Could you check a few things on this model? Use its own coordinates, in mm. A direction names the side the tool comes from. Give positions to 0.01 mm unless a question says otherwise; leave off trailing zeros. Write each loop counter-clockwise with the first axis right and the second up, starting at its lowest first coordinate (ties: lowest second). Pieces come first, ordered by that corner, then holes. Notation, with made-up numbers: M -19.5,26 L 13.5,26 A22 cw 13.5,48 Z; hole C 63,46.25 d11. An arc over 180 degrees is marked long. Use one line per item in the form item = value.
from build123d import *

# Parameters (mm, degrees)
SKETCH1_W           = 22.86
SKETCH1_H           = 22.86
BOSS_EXTRUDE1_DEPTH = 1.27
SKETCH3_W           = 22.86
SKETCH3_H           = 1.27
BOSS_EXTRUDE2_DEPTH = 47.593039283
SKETCH4_R           = 4
CUT_EXTRUDE2_DEPTH  = 10
SKETCH5_R           = 4
SKETCH5_W           = 8
SKETCH5_H           = 10.275395712
CUT_EXTRUDE3_DEPTH  = 2.54
SCALE2_SCALE        = 2.1


with BuildPart() as part:
    # Sketch1 → Boss-Extrude1 (new body)
    with BuildSketch(Plane(origin=(0, 0, 0), x_dir=(1, 0, 0), z_dir=(0, 1, 0))):
        with Locations((0.164586144, 0.124003255)):
            Rectangle(SKETCH1_W, SKETCH1_H)
    extrude(amount=BOSS_EXTRUDE1_DEPTH)

    # Sketch3 → Boss-Extrude2 (add)
    with BuildSketch(Plane.XZ):
        with Locations((0.164586144, -10.919003255)):
            Rectangle(SKETCH3_W, SKETCH3_H)
    extrude(amount=-BOSS_EXTRUDE2_DEPTH)

    # Sketch4 → Cut-Extrude2 (cut)
    with BuildSketch(Plane(origin=(0, 1.27, 0), x_dir=(1, 0, 0), z_dir=(0, 1, 0))):
        with Locations(Location((0, 0, 0), (0, 0, 270))):
            Circle(SKETCH4_R)
    extrude(amount=-CUT_EXTRUDE2_DEPTH, mode=Mode.SUBTRACT)

    # Sketch5 → Cut-Extrude3 (cut)
    with BuildSketch(Plane.XY.offset(-10.284003255)):
        with Locations((0.082545716, 37.799520725)):
            Circle(SKETCH5_R)
        with Locations((0.034649226, 27.524125013)):
            Circle(SKETCH5_R)
        with Locations((0.082545716, 32.661822869)):
            Rectangle(SKETCH5_W, SKETCH5_H)
        with BuildLine():
            ThreePointArc((4.034649226, 27.524125013), (0.344153636, 31.512132914), (-3.917454284, 28.141278028))
            Line((-3.917454284, 28.141278028), (-3.917454284, 27.524125013))
            Line((-3.917454284, 27.524125013), (4.034649226, 27.524125013))
        make_face()
        with BuildLine():
            Line((-3.917454284, 27.524125013), (-3.917454284, 28.141278028))
            ThreePointArc((-3.917454284, 28.141278028), (-0.274855184, 23.536117112), (4.034649226, 27.524125013))
            Line((4.034649226, 27.524125013), (-3.917454284, 27.524125013))
        make_face()
        with Locations((0, 10.961912138)):
            Circle(SKETCH5_R)
        with BuildLine():
            ThreePointArc((4.082545716, 37.799520725), (0.082545716, 41.799520725), (-3.917454284, 37.799520725))
            Line((-3.917454284, 37.799520725), (4.082545716, 37.799520725))
        make_face()
        with BuildLine():
            Line((4.082545716, 37.799520725), (-3.917454284, 37.799520725))
            ThreePointArc((-3.917454284, 37.799520725), (0.082545716, 33.799520725), (4.082545716, 37.799520725))
        make_face()
    extrude(amount=-CUT_EXTRUDE3_DEPTH, mode=Mode.SUBTRACT)


with BuildPart() as part_1:
    # Scale2: scaled about (0, 0, 0)
    add(part.part.scale(SCALE2_SCALE))


solid = part_1.part
1) If I drill on L1, parallel to Y at x = 0, z = -23; L2, parallel to X at y = 0.85, z = 0; L3, parallel to Z at x = 9.5, y = 9, over which ranges is the centre line in solid material (lowest first)?
Checked values:
L1 = 0 to 14.62, 31.42 to 49.4, 87.78 to 99.95
L2 = -23.66 to -8.4, 8.4 to 24.35
L3 = -24.26 to -21.6
2) For faces 1 (the flat face through (-8.227, 69, -23)), 2 (the flat face through (5.3, 50.6, -21.596)), 3 (the flat face through (0, 1, 23.743)), which set-ups out of +Z, -Z, +X, -X, +Y, -Y let a thin tool reach every point of the face, with its end or its side?
Checked values:
face_1 = +Z, -Z
face_2 = +Z, +X, -X, +Y
face_3 = +Z, +X, -X, +Y, -Y
3) I want a section at D-D, the plane x = -15.5. Please give me the cut outline in (y, z).
Checked values:
outline = M 0,-24.26 L 99.95,-24.26 L 99.95,-21.6 L 2.67,-21.6 L 2.67,23.74 L 0,23.74 Z
4) I want a section at C-C, the plane x = 0. Please give me the cut outline in (y, z), plus the area to 3 significant figures.
Checked values:
outline = M 0,-24.26 L 14.62,-24.26 L 14.62,-21.6 L 2.67,-21.6 L 2.67,-8.4 L 0,-8.4 Z; M 0,8.4 L 2.67,8.4 L 2.67,23.74 L 0,23.74 Z; M 31.42,-24.26 L 49.4,-24.26 L 49.4,-21.6 L 31.42,-21.6 Z; M 87.78,-24.26 L 99.95,-24.26 L 99.95,-21.6 L 87.78,-21.6 Z
area = 196 mm2
5) For pin 1 Ø10 at (x, z) = (-15, -9) entering from +Y; pin 2 Ø6 at (x, y) = (5.5, 71.5) entering from -Z; pin 3 Ø24 at (x, y) = (3, 48.5) entering from +Z, each with a flat end and sliding along its axis, tell me the tip position at first contact or that it passes through.
Checked values:
pin_1 = 2.67
pin_2 = through
pin_3 = -21.6
6) Thinking about a two-plate mould opening in Y: for faces 4 (the flat face through (0, 2.667, -9)), 5 (the cylindrical face through (2.523, 1.352, 8.012)), 6 (the cylindrical face through (-0.77, 49.443, -22.911)), which applies, released by +Y, released by -Y, zero draft, split by the parting line, or undercut?
Checked values:
face_4 = released by +Y
face_5 = zero draft
face_6 = undercut
7) I want a section at A-A, the plane z = 0. Please give me the cut outline in (x, y).
Checked values:
outline = M -23.66,0 L -8.4,0 L -8.4,2.67 L -23.66,2.67 Z; M 8.4,0 L 24.35,0 L 24.35,2.67 L 8.4,2.67 Z
8) I want a section at B-B, the plane y = 71.5. Please give me the cut outline in (x, z), plus the area to 3 significant figures.
Checked values:
outline = M -23.66,-24.26 L -8.23,-24.26 L -8.23,-21.6 L -23.66,-21.6 Z; M 8.57,-24.26 L 24.35,-24.26 L 24.35,-21.6 L 8.57,-21.6 Z
area = 83.2 mm2
